from build123d import *

# Parameters (mm, degrees)
BOSS_EXTRUDE1_DEPTH        = 100
SKETCH2_R                  = 3
CUT_EXTRUDE1_DEPTH         = 4.5
SKETCH3_R                  = 1.75
CUT_EXTRUDE2_DEPTH         = 101.202295383
CHAMFER1_SIZE              = 0.2
LPATTERN1_COUNT            = 5
LPATTERN1_PITCH            = 20
CHAMFER1_OF_LPATTERN1_SIZE = 0.2


with BuildPart() as part:
    # Sketch1 → Boss-Extrude1 (new body)
    with BuildSketch(Plane.XY):
        with BuildLine():
            Line((4.5, -2.5), (4.5, 0.514709157))
            ThreePointArc((4.5, 0.514709157), (4.188868575, 0.667088042), (3.988911299, 0.95))
            Line((3.988911299, 0.95), (3.35, 0.95))
            ThreePointArc((3.35, 0.95), (3.1, 1.2), (3.35, 1.45))
            Line((3.35, 1.45), (3.988911299, 1.45))
            ThreePointArc((3.988911299, 1.45), (4.188868575, 1.732911958), (4.5, 1.885290843))
            Line((4.5, 1.885290843), (4.5, 2.5))
            Line((4.5, 2.5), (4, 3))
            Line((4, 3), (-4, 3))
            Line((-4, 3), (-4.5, 2.5))
            Line((-4.5, 2.5), (-4.5, 1.885290843))
            ThreePointArc((-4.5, 1.885290843), (-4.188868575, 1.732911958), (-3.988911299, 1.45))
            Line((-3.988911299, 1.45), (-3.35, 1.45))
            ThreePointArc((-3.35, 1.45), (-3.1, 1.2), (-3.35, 0.95))
            Line((-3.35, 0.95), (-3.988911299, 0.95))
            ThreePointArc((-3.988911299, 0.95), (-4.188868575, 0.667088042), (-4.5, 0.514709157))
            Line((-4.5, 0.514709157), (-4.5, -2.5))
            Line((-4.5, -2.5), (-4, -3))
            Line((-4, -3), (4, -3))
            Line((4, -3), (4.5, -2.5))
        make_face()
    extrude(amount=BOSS_EXTRUDE1_DEPTH)

    # Sketch2 → Cut-Extrude1 (cut)
    with BuildSketch(Plane(origin=(0, 3, 0), x_dir=(1, 0, 0), z_dir=(0, 1, 0))):
        with Locations(Location((0, -10, 0), (0, 0, 180))):
            Circle(SKETCH2_R)
    cut_extrude1 = extrude(amount=-CUT_EXTRUDE1_DEPTH, mode=Mode.SUBTRACT)

    # Sketch3 → Cut-Extrude2 (cut, through all)
    with BuildSketch(Plane(origin=(0, -1.5, 0), x_dir=(1, 0, 0), z_dir=(0, 1, 0))):
        with Locations(Location((0, -10, 0), (0, 0, 180))):
            Circle(SKETCH3_R)
    cut_extrude2 = extrude(amount=-CUT_EXTRUDE2_DEPTH, mode=Mode.SUBTRACT)

    # Chamfer1
    chamfer1_edges = [part.edges().sort_by_distance(p)[0] for p in [
        (3, 3, 10),
        (1.75, -3, 10),
    ]]
    chamfer(chamfer1_edges, length=CHAMFER1_SIZE)

    # LPattern1: Cut-Extrude1, Cut-Extrude2 ×5
    with Locations(*[(0, 0, i * LPATTERN1_PITCH) for i in range(1, LPATTERN1_COUNT)]):
        add(cut_extrude1, mode=Mode.SUBTRACT)
        add(cut_extrude2, mode=Mode.SUBTRACT)

    # Chamfer1 of LPattern1
    chamfer1_of_lpattern1_edges = [part.edges().sort_by_distance(p)[0] for p in [
        (3, 3, 30),
        (1.75, -3, 30),
        (3, 3, 50),
        (1.75, -3, 50),
        (3, 3, 70),
        (1.75, -3, 70),
        (3, 3, 90),
        (1.75, -3, 90),
    ]]
    chamfer(chamfer1_of_lpattern1_edges, length=CHAMFER1_OF_LPATTERN1_SIZE)


solid = part.part
Source: CAD feature listing. Evaluate the final solid. Frame: model axes, mm. A direction names the side the tool comes from. Round coordinates to 2 decimals unless told otherwise and drop trailing zeros. Order: outer loops, then holes, each group sorted by start corner. A loop starts at its lowest first (then second) coordinate and runs counter-clockwise, first axis right, second up. Notation, with made-up numbers: (57.25, 84) - (95.25, 84) arc R23 cw to (95.25, 95) - close; hole circle Ø8 at (24.5, 12.25). An arc over 180 degrees is marked (long way). Use a Markdown table: item, result. Add a question column.
1. Line query: probe 1 along Z at (x, y) = (0, -2); probe 2 along Y at (x, z) = (3.25, 87); probe 3 along Z at (x, y) = (0, -0.2). Output: solid intervals per line, ascending.
2. Set-up query: faces 4 (the cylindrical face through (-0.9, -2.1, 91.5)), 5 (the flat face through (-2, -1.5, 70)). Return all of +Z, -Z, +X, -X, +Y, -Y with unobstructed straight access to the full face (end or side cutting, diameter ignored); none if empty.
3. First-contact query: pin 1 (5 mm diameter, centred on x = 0, z = 90, fed in from +Y); pin 2 (1.8 mm diameter, centred on x = 0, z = 70.5, fed in from +Y). Flat tips, straight axial feed; report the tip coordinate or a pass-through.
4. Section query B-B (z = 19.5). Return the cut outline in (x, y).
5. Mould query, pull axis X, two halves, no side actions, for faces 1 (the flat face through (4.5, -1, 49)), 2 (the flat face through (0, -1.5, 28)), 3 (the flat face through (-4.5, -1, 49)). Classes: +X half, -X half, draft (parallel to the pull), parting line (faces both ways), or undercut.
6. Section query C-C (x = 0). Give the number of separate pieces and of enclosed holes in the cut face, then the cut area to 3 significant figures.
Derived:
| question | item | result |
|---|---|---|
| 1 | probe 1 | 0 to 8.25, 11.75 to 28.25, 31.75 to 48.25, 51.75 to 68.25, 71.75 to 88.25, 91.75 to 100 |
| 1 | probe 2 | -3 to 0.97, 1.43 to 3 |
| 1 | probe 3 | 0 to 7, 13 to 27, 33 to 47, 53 to 67, 73 to 87, 93 to 100 |
| 2 | face 4 | +Y, -Y |
| 2 | face 5 | +Y |
| 3 | pin 1 | y = -1.5 |
| 3 | pin 2 | through |
| 4 | outline | (-4.5, -2.5) - (-4, -3) - (4, -3) - (4.5, -2.5) - (4.5, 0.51) arc R0.7 cw to (3.99, 0.95) - (3.35, 0.95) arc R0.25 cw to (3.35, 1.45) - (3.99, 1.45) arc R0.7 cw to (4.5, 1.89) - (4.5, 2.5) - (4, 3) - (-4, 3) - (-4.5, 2.5) - (-4.5, 1.89) arc R0.7 cw to (-3.99, 1.45) - (-3.35, 1.45) arc R0.25 cw to (-3.35, 0.95) - (-3.99, 0.95) arc R0.7 cw to (-4.5, 0.51) - close |
| 5 | face 1 | +X half |
| 5 | face 2 | undercut |
| 5 | face 3 | -X half |
| 6 | separate pieces | 6 |
| 6 | enclosed holes | 0 |
| 6 | area | 438 mm2 |
